Input: dimensioned drawing with shaded views. Units: mm. Origin: part minimum x, y, z. Round coordinates to 2 decimals unless told otherwise and drop trailing zeros. Loops run counter-clockwise (first coordinate to the right, second up) from the corner with the lowest first, then second, coordinate; pieces in that order, holes last. Notation, with made-up numbers: M -33,34.5 L 25,34.5 A10 ccw 25,43.5 Z; hole C 36.25,84 d8. An arc over 180 degrees is marked long. Write each question's results on one line, items separated by ' | '. Start each with the question number.
1. Contact query for flat-ended pins moving along their axis: pin 1 Ø6 at (y, z) = (4, 8) entering from -X; pin 2 Ø5 at (y, z) = (9.5, 8.5) entering from -X; pin 3 Ø4 at (y, z) = (4, 2) entering from -X; pin 4 Ø6 at (y, z) = (14, 5.5) entering from -X. Output: stop coordinate, or through.
2. Section A-A on z = 6.25. Output: boundary loops of the cut face in (x, y).
3. Ray query, line 1 (X direction, y = 8.25, z = 5); line 2 (X direction, y = 9, z = 6); line 3 (Y direction, x = 6.5, z = 2.5). Return the intervals inside material, ascending.
4. Section C-C on y = 12. Output: boundary loops of the cut face in (x, z).
5. Section B-B on x = 7. Output: boundary loops of the cut face in (y, z), and give its area (3 significant figures).
6. Section D-D on x = 50.5. Output: boundary loops of the cut face in (y, z), and give its area (3 significant figures).
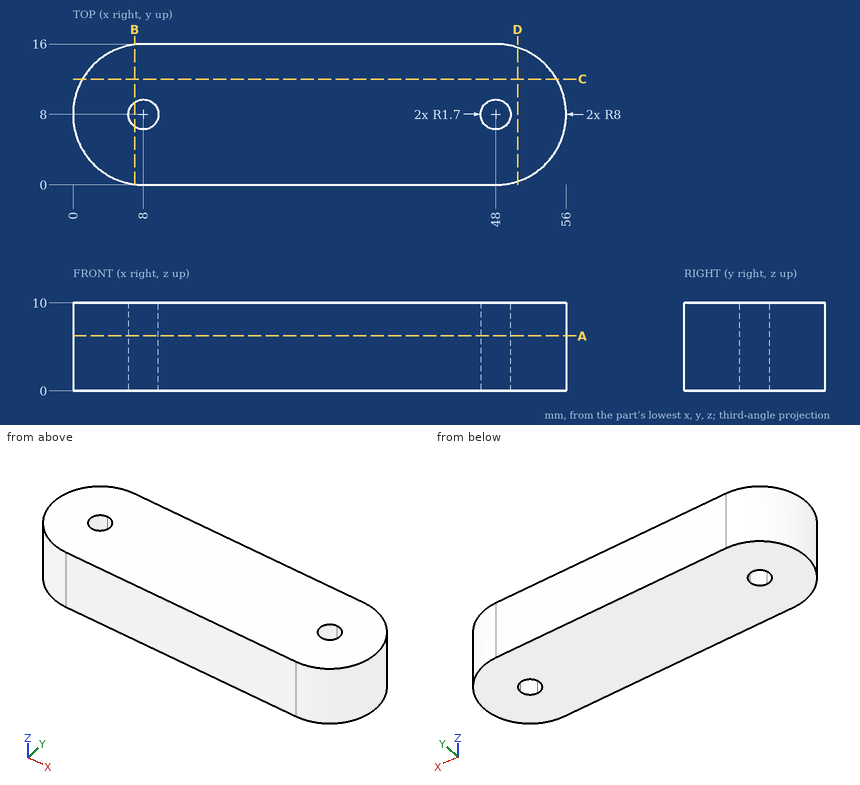
Taken from the geometry:
1) pin 1: x = 0.06 | pin 2: x = 0 | pin 3: x = 0.25 | pin 4: x = 0.58
2) outline: M 8,0 L 48,0 A8 ccw 48,16 L 8,16 A8 ccw Z; hole M 8,6.3 A1.7 ccw 9.7,8 A1.7 ccw 8,9.7 A1.7 ccw Z; hole M 48,6.3 A1.7 ccw 49.7,8 A1.7 ccw 48,9.7 A1.7 ccw Z
3) line 1: 0 to 6.32, 9.68 to 46.32, 49.68 to 56 | line 2: 0.06 to 6.63, 9.37 to 46.63, 49.37 to 55.94 | line 3: 0.14 to 7.2, 8.8 to 15.86
4) outline: M 1.07,0 L 54.93,0 L 54.93,10 L 1.07,10 Z
5) outline: M 0.06,0 L 6.63,0 L 6.63,10 L 0.06,10 Z; M 9.37,0 L 15.94,0 L 15.94,10 L 9.37,10 Z | area: 131 mm^2
6) outline: M 0.4,0 L 15.6,0 L 15.6,10 L 0.4,10 Z | area: 152 mm^2
